Build history of the part. All positions in model axes, mm. Face numbers are marked on the shaded views. A direction names the side the tool comes from. Round coordinates to 2 decimals unless told otherwise and drop trailing zeros. Loops run counter-clockwise (first coordinate to the right, second up) from the corner with the lowest first, then second, coordinate; pieces in that order, holes last. Notation, with made-up numbers: (-8.5, -14) -> (5.5, -14) arc R23 ccw to (5.5, 17) -> close; hole circle Ø10 at (-30.75, 83.5). An arc over 180 degrees is marked (long way). Put each result on its own line as item: value. Start each with the question number.
```python
from build123d import *

# Parameters (mm, degrees)
F1_DEPTH       = 2.54
F3_DEPTH       = 36.322
F4_W           = 2.5400000004
F4_H           = 53.594
F4_W_2         = 2.5400000003
F4_H_2         = 51.054
F5_DEPTH       = 7.62
F6_R           = 2.032
F7_SIZE        = 5.08
F8_SIZE        = 5.08
F10_DEPTH      = 31.9278
F12_R          = 1.778
F13_DEPTH      = 2.54
F14_SIZE       = 5.08
F16_DEPTH      = 2.54
F16_DEPTH_BACK = 25.4


with BuildPart() as f1:
    # F0 (on Front) → F1 (new body)
    with BuildSketch(Plane.XZ):
        Polygon((18.161, 9.3117938122), (18.161, 30.607), (-18.161, 30.607), (-18.161, 9.3117938122), (-18.161, -9.3117938122), (-18.161, -30.607), (18.161, -30.607), (18.161, -9.3117938122), align=None)
    extrude(amount=F1_DEPTH)

    # F2 (on face) → F3 (join, through all)
    with BuildSketch(Plane.YZ.offset(18.161)):
        Polygon((-2.54, 28.067), (-2.54, 30.607), (-34.4678, 30.607), (-34.4678, -30.607), (-31.9278, -30.607), (-31.9278, -26.035), (-31.9278, 28.067), align=None)
        with BuildLine():
            ThreePointArc((-31.9278, -30.607), (-29.6418, -28.321), (-31.9278, -26.035))
            Line((-31.9278, -26.035), (-31.9278, -30.607))
        make_face()
    extrude(amount=-F3_DEPTH)

    # F4 (on face) → F5 (join)
    with BuildSketch(Plane.XZ.offset(2.54)):
        with Locations((-16.8910000002, 1.27)):
            Rectangle(F4_W, F4_H)
        with Locations((16.8909999998, 2.54)):
            Rectangle(F4_W_2, F4_H_2)
    extrude(amount=F5_DEPTH)

    # F6
    f6_edges = [f1.edges().sort_by_distance(p)[0] for p in [
        (0, -31.9278, -30.607),
        (0, -31.9278, -26.035),
    ]]
    fillet(f6_edges, radius=F6_R)

    # F7
    f7_edges = [f1.edges().sort_by_distance(p)[0] for p in [
        (18.161, -34.4678, 0),
    ]]
    chamfer(f7_edges, length=F7_SIZE)

    # F8
    f8_edges = [f1.edges().sort_by_distance(p)[0] for p in [
        (-18.161, -34.4678, 0),
    ]]
    chamfer(f8_edges, length=F8_SIZE)

    # F9 (on face) → F10 (cut, through all)
    with BuildSketch(Plane.XZ.offset(34.4678)):
        with BuildLine():
            ThreePointArc((-15.621, -24.511), (-15.910574375, -25.556455375), (-16.6967647059, -26.3039411765))
            ThreePointArc((-16.6967647059, -26.3039411765), (-17.8387457553, -28.8754364388), (-15.621, -30.607))
            Line((-15.621, -30.607), (-15.621, -24.511))
        make_face()
        with BuildLine():
            ThreePointArc((15.621, -30.607), (17.8387457553, -28.8754364388), (16.6967647059, -26.3039411765))
            ThreePointArc((16.6967647059, -26.3039411765), (15.910574375, -25.556455375), (15.621, -24.511))
            Line((15.621, -24.511), (15.621, -30.607))
        make_face()
    extrude(amount=-F10_DEPTH, mode=Mode.SUBTRACT)

    # F12 (on face) → F13 (join, through all)
    with BuildSketch(Plane(origin=(0, 0, 0), x_dir=(-1, 0, 0), z_dir=(0, 1, 0))):
        with BuildLine():
            Line((-7.493, 38.1), (-7.493, 30.607))
            Line((-7.493, 30.607), (7.493, 30.607))
            Line((7.493, 30.607), (7.493, 38.1))
            ThreePointArc((7.493, 38.1), (0, 45.593), (-7.493, 38.1))
        make_face()
        with Locations((0, 38.1)):
            Circle(F12_R, mode=Mode.SUBTRACT)
        with BuildLine():
            Line((-6.35, -30.607), (-7.493, -30.607))
            Line((-7.493, -30.607), (-7.493, -38.1))
            ThreePointArc((-7.493, -38.1), (0, -45.593), (7.493, -38.1))
            Line((7.493, -38.1), (7.493, -30.607))
            Line((7.493, -30.607), (6.35, -30.607))
            Line((6.35, -30.607), (0, -30.607))
            Line((0, -30.607), (-6.35, -30.607))
        make_face()
        with Locations((0, -38.1)):
            Circle(F12_R, mode=Mode.SUBTRACT)
    extrude(amount=-F13_DEPTH)

    # F14
    f14_edges = [f1.edges().sort_by_distance(p)[0] for p in [
        (-7.493, -1.27, -30.607),
        (7.493, -1.27, -30.607),
        (7.493, -1.27, 30.607),
        (-7.493, -1.27, 30.607),
    ]]
    chamfer(f14_edges, length=F14_SIZE)

    # F15 (on face) → F16 (cut, two sides)
    with BuildSketch(Plane(origin=(0, 0, 28.067), x_dir=(1, 0, 0), z_dir=(0, 0, -1))) as f16_sk:
        Polygon((5.715, 27.3558), (0, 27.3558), (-5.715, 27.3558), (-5.715, 19.7358), (5.715, 19.7358), align=None)
    extrude(amount=-F16_DEPTH, mode=Mode.SUBTRACT)
    extrude(f16_sk.sketch, amount=F16_DEPTH_BACK, mode=Mode.SUBTRACT)


solid = f1.part
```
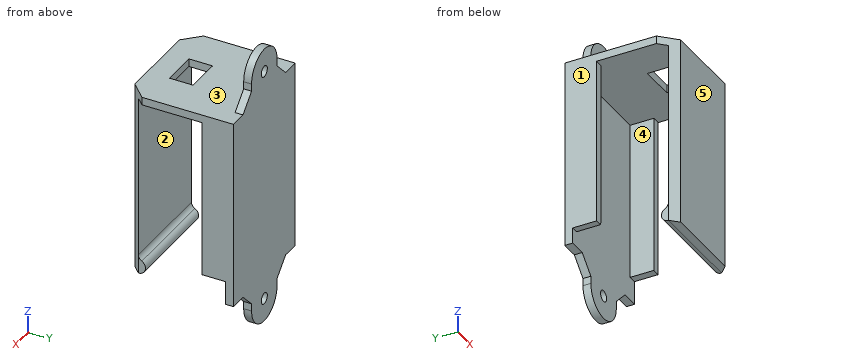
Item 1: 3-axis set-ups, long thin cutter, end or side, ignore diameter. For the marked faces 4 and 5: which of +Z, -Z, +X, -X, +Y, -Y reach the whole face in a straight line?
Item 2: Cut at B-B on z = 8.5. Write the cut outline in (x, y), then the cut area to 3 significant figures.
Item 3: Wall check: line 1 (Z direction, x = 0, y = -1); line 2 (Y direction, x = 12.5, z = -7); line 3 (X direction, y = -1, z = 38). Give the ranges that are in metal, low to high. Write a range as from..to.
Item 4: Drop flat-ended pins along their axis: pin 1 (0.7 mm diameter, centred on y = -1.5, z = -37, fed in from -X); pin 2 (1.1 mm diameter, centred on y = -30.5, z = -26, fed in from -X); pin 3 (3 mm diameter, centred on x = -7.5, y = -19.5, fed in from -Z). Give the stop position or say it passes through.
Item 5: Cut at C-C on y = -8. Write the cut outline in (x, z).
Item 6: Cut at A-A on x = 0. Write the cut outline in (y, z), then the cut area to 3 significant figures.
Item 7: Pull direction Z, two halves, no side cores. Call the marked faces 1, 2 and 3: +Z half, -Z half, draft (parallel to the pull), parting line (faces both ways), or undercut.
Ans:
1. face 4: -Z
1. face 5: +Z, -Z, +X, -X, -Y
2. outline: (-18.16, -10.16) -> (-15.62, -10.16) -> (-15.62, -2.54) -> (15.62, -2.54) -> (15.62, -10.16) -> (18.16, -10.16) -> (18.16, 0) -> (-18.16, 0) -> close; (-15.62, -31.93) -> (-13.08, -34.47) -> (13.08, -34.47) -> (15.62, -31.93) -> close
2. area: 204 mm2
3. line 1: z = -45.59..-39.88, -36.32..36.32, 39.88..45.59
3. line 2: y = -34.47..-31.93, -2.54..0
3. line 3: x = -7.49..-1.78, 1.78..7.49
4. pin 1: stops at x = -7.49
4. pin 2: stops at x = -15.62
4. pin 3: stops at z = 28.07
5. outline: (-18.16, -25.53) -> (-15.89, -25.53) arc R2.03 ccw to (-15.62, -24.51) -> (-15.62, 28.07) -> (15.62, 28.07) -> (15.62, -22.99) -> (18.16, -22.99) -> (18.16, 30.61) -> (-18.16, 30.61) -> close
6. outline: (-34.47, -30.61) -> (-31.93, -30.61) arc R2.29 ccw to (-30.85, -26.3) arc R2.03 cw to (-31.93, -24.51) -> (-31.93, 28.07) -> (-27.36, 28.07) -> (-27.36, 30.61) -> (-34.47, 30.61) -> close; (-19.74, 28.07) -> (-2.54, 28.07) -> (-2.54, -36.32) -> (0, -36.32) -> (0, 36.32) -> (-2.54, 36.32) -> (-2.54, 30.61) -> (-19.74, 30.61) -> close; (-2.54, -45.59) -> (0, -45.59) -> (0, -39.88) -> (-2.54, -39.88) -> close; (-2.54, 39.88) -> (0, 39.88) -> (0, 45.59) -> (-2.54, 45.59) -> close
6. area: 433 mm2
7. face 1: draft
7. face 2: undercut
7. face 3: +Z half
